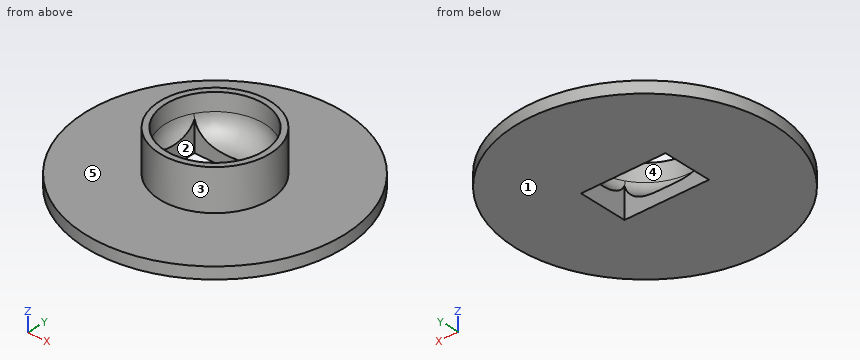
```python
from build123d import *

# Parameters (mm, degrees)
F0_R     = 11
F0_W     = 7.2
F0_H     = 4.2
F1_DEPTH = 1
F2_R     = 4.7
F2_R_2   = 4.2
F3_DEPTH = 3.5


# Not quite as in the source:
# - a fillet or chamfer that OpenCascade refuses, or shapes differently, is made with other operations: its cross-section is extruded or revolved along the edge and cut away or added


with BuildPart() as f1:
    # F0 (on Top) → F1 (new body)
    with BuildSketch(Plane.XY):
        Circle(F0_R)
        Rectangle(F0_W, F0_H, mode=Mode.SUBTRACT)
    extrude(amount=F1_DEPTH)

    # F2 (on face) → F3 (join)
    with BuildSketch(Plane.XY.offset(1)):
        Circle(F2_R)
        Circle(F2_R_2, mode=Mode.SUBTRACT)
    extrude(amount=F3_DEPTH)

    # F4: fillet of radius 2 on 1 edges, made by hand


with BuildPart() as f4_tool2:
    # F4_s3 → F4_t4 (revolve)
    with BuildSketch(Plane.XZ):
        with BuildLine():
            ThreePointArc((2.2, 1), (3.6142135624, 1.5857864376), (4.2, 3))
            Line((4.2, 3), (4.2, 1))
            Line((4.2, 1), (2.2, 1))
        make_face()
    revolve(axis=Axis((0, 0, 1), (0, 0, 1)))

    split(bisect_by=Plane.YZ.offset(3.6), keep=Keep.TOP)


with BuildPart() as f1_1:
    add(f1.part)

    # F4_t1: union F4_tool2
    add(f4_tool2.part)


with BuildPart() as f4_tool7:
    # F4_s8 → F4_t9 (revolve)
    with BuildSketch(Plane.XZ):
        with BuildLine():
            ThreePointArc((2.2, 1), (3.6142135624, 1.5857864376), (4.2, 3))
            Line((4.2, 3), (4.2, 1))
            Line((4.2, 1), (2.2, 1))
        make_face()
    revolve(axis=Axis((0, 0, 1), (0, 0, 1)))

    split(bisect_by=Plane.XZ.offset(-2.1), keep=Keep.BOTTOM)


with BuildPart() as f1_2:
    add(f1_1.part)

    # F4_t6: union F4_tool7
    add(f4_tool7.part)


with BuildPart() as f4_tool12:
    # F4_s13 → F4_t14 (revolve)
    with BuildSketch(Plane.XZ):
        with BuildLine():
            ThreePointArc((2.2, 1), (3.6142135624, 1.5857864376), (4.2, 3))
            Line((4.2, 3), (4.2, 1))
            Line((4.2, 1), (2.2, 1))
        make_face()
    revolve(axis=Axis((0, 0, 1), (0, 0, 1)))

    split(bisect_by=Plane.XZ.offset(2.1), keep=Keep.TOP)


with BuildPart() as f1_3:
    add(f1_2.part)

    # F4_t11: union F4_tool12
    add(f4_tool12.part)


with BuildPart() as f4_tool17:
    # F4_s18 → F4_t19 (revolve)
    with BuildSketch(Plane.XZ):
        with BuildLine():
            ThreePointArc((2.2, 1), (3.6142135624, 1.5857864376), (4.2, 3))
            Line((4.2, 3), (4.2, 1))
            Line((4.2, 1), (2.2, 1))
        make_face()
    revolve(axis=Axis((0, 0, 1), (0, 0, 1)))

    split(bisect_by=Plane.YZ.offset(-3.6), keep=Keep.BOTTOM)


with BuildPart() as f1_4:
    add(f1_3.part)

    # F4_t16: union F4_tool17
    add(f4_tool17.part)


solid = f1_4.part
```
CAD build for the part. Positions are in the model's coordinates, mm. Face numbers are marked on the shaded views. A direction names the side the tool comes from. Coordinates: 2 decimals unless noted, no trailing zeros. Order: outer loops, then holes, each group sorted by start corner. A loop starts at its lowest first (then second) coordinate and runs counter-clockwise, first axis right, second up. Notation, with made-up numbers: M 21.5,37 L 54.5,37 A26 cw 54.5,63 Z; hole C 30.25,2 d8. An arc over 180 degrees is marked long. Write each question's results on one line, items separated by ' | '. Start each with the question number.
Q1. Cut at A-A (y = 0). List the corners of the cut face in (x, z).
Q2. Pull direction Y, two halves, no side cores. Call the marked faces 3, 4 and 5: +Y half, -Y half, draft (parallel to the pull), parting line (faces both ways), or undercut.
Q3. Flat gauge pins, fed straight in: P1, Ø1, axis at x = -4, z = 3.5, coming from the -Y side; P2, Ø1.5, axis at x = 3.5, z = 3, coming from the -Y side; P3, Ø2, axis at y = 5, z = 1.5, coming from the -X side. Where does each tip first touch, or does it go through?
Q4. Cut at C-C (y = 5). List the corners of the cut face in (x, z), then the cut area to 3 significant figures.
Q5. Which spindle directions (+Z, -Z, +X, -X, +Y, -Y) get a long thin tool onto all of the face, cutting with end or side? Do the marked faces 1 and 2. Say none if no direction does.
Q6. Cut at D-D (y = -8.75). List the corners of the cut face in (x, z), then the cut area to 3 significant figures.
Q7. Cut at B-B (x = 0). List the corners of the cut face in (y, z).
Q8. Drill centre lines: probe 1 along Y at (x, z) = (0, 3.85); probe 2 along Y at (x, z) = (-1.5, 2.35); probe 3 along X at (y, z) = (3, 2.65). Where is each one in solid material? Low to high. Write a range as from..to.
Found:
1) outline: M -11,0 L -3.6,0 L -3.6,1.57 A2 cw -4.2,3 L -4.2,4.5 L -4.7,4.5 L -4.7,1 L -11,1 Z; M 3.6,0 L 11,0 L 11,1 L 4.7,1 L 4.7,4.5 L 4.2,4.5 L 4.2,3 A2 cw 3.6,1.57 Z
2) face 3: parting line | face 4: undercut | face 5: draft
3) P1: y = -3.14 | P2: y = -3.81 | P3: x = -10.19
4) outline: M -9.8,0 L 9.8,0 L 9.8,1 L -9.8,1 Z | area: 19.6 mm²
5) face 1: -Z, +X, -X, +Y, -Y | face 2: +Z, -Z
6) outline: M -6.67,0 L 6.67,0 L 6.67,1 L -6.67,1 Z | area: 13.3 mm²
7) outline: M -11,0 L -2.1,0 L -2.1,1 L -2.2,1 A2 cw -4.2,3 L -4.2,4.5 L -4.7,4.5 L -4.7,1 L -11,1 Z; M 2.1,0 L 11,0 L 11,1 L 4.7,1 L 4.7,4.5 L 4.2,4.5 L 4.2,3 A2 cw 2.2,1 L 2.1,1 Z
8) probe 1: -4.7..-4.2, 4.2..4.7 | probe 2: -4.45..-3.81, 3.81..4.45 | probe 3: -3.62..-2.9, 2.9..3.62
